For this review, take the finished solid that the model builds, in its own axes (mm). Face numbers are marked on the shaded views. Round coordinates to 2 decimals unless told otherwise and drop trailing zeros. Loops run counter-clockwise (first coordinate to the right, second up) from the corner with the lowest first, then second, coordinate; pieces in that order, holes last.
1. Consider section C-C on x = -25. State the section outline as (y, z) points.
2. Consider section D-D on y = 0.4. State the section outline as (x, z) points.
3. To check wall thickness, follow line 1 along Z through (x, y) = (-12.25, 2.3); line 2 along X through (y, z) = (1.45, -5); line 3 along Y through (x, z) = (-22.25, -6.5). State the ranges of each line that lie inside material, in increasing order.
4. Consider section B-B on z = 9.5. State the section outline as (x, y) points.
5. Consider section A-A on y = 1.7. State the section outline as (x, z) points, then the cut area to 3 significant figures.
6. Draft analysis for pull direction X (two halves, no side actions). For the marked faces 1, 2, 3 and 4, state which applies: released by +X, released by -X, zero draft, split by the parting line, or undercut.
7. Clearance check with flat-ended pins moving along their axes: pin 1 Ø2 at (x, z) = (-14.5, 2) entering from +Y; pin 2 Ø1.1 at (x, y) = (-19.5, 0.5) entering from +Z. State where each tip first meets the part, or that it passes through.
from build123d import *

# Parameters (mm, degrees)
MAIN_BOARD_OUTLINE_W = 18.5
MAIN_BOARD_OUTLINE_H = 28
SIDE1_DEPTH          = 1
SKETCH2_W            = 2
SKETCH2_H            = 28
WALLS_DEPTH          = 2.3
SKETCH3_R            = 1.5
SCREW_HOLE_DEPTH     = 2.3
SKETCH4_W            = 4.6228
SKETCH4_H            = 2
SPI_HOLE_DEPTH       = 2.3
SKETCH5_W            = 2
SKETCH5_H            = 4
CUT_EXTRUDE3_DEPTH   = 2.3


with BuildPart() as part:
    # main board outline → side1 (new body)
    with BuildSketch(Plane(origin=(0, 0, 0), x_dir=(1, 0, 0), z_dir=(0, 1, 0))):
        with Locations((-19.997374583, 0.651042113)):
            Rectangle(MAIN_BOARD_OUTLINE_W, MAIN_BOARD_OUTLINE_H)
    extrude(amount=SIDE1_DEPTH)

    # Sketch2 → walls (add)
    with BuildSketch(Plane(origin=(0, 1, 0), x_dir=(1, 0, 0), z_dir=(0, 1, 0))):
        with Locations((-28.247374583, 0.651042113)):
            Rectangle(SKETCH2_W, SKETCH2_H)
        with Locations((-11.747374583, 0.651042113)):
            Rectangle(SKETCH2_W, SKETCH2_H)
    extrude(amount=WALLS_DEPTH)

    # Sketch3 → screw hole (cut)
    with BuildSketch(Plane(origin=(0, 0, 0), x_dir=(-1, 0, 0), z_dir=(0, -1, 0))):
        with Locations((24.504374583, -10.605757887)):
            Circle(SKETCH3_R)
    extrude(amount=-SCREW_HOLE_DEPTH, mode=Mode.SUBTRACT)

    # Sketch4 → spi hole (cut)
    with BuildSketch(Plane(origin=(0, 0, 0), x_dir=(-1, 0, 0), z_dir=(0, -1, 0))):
        with Locations((18.687974583, -12.348957887)):
            Rectangle(SKETCH4_W, SKETCH4_H)
    extrude(amount=-SPI_HOLE_DEPTH, mode=Mode.SUBTRACT)

    # Sketch5 → Cut-Extrude3 (cut)
    with BuildSketch(Plane(origin=(0, 3.3, 0), x_dir=(1, 0, 0), z_dir=(0, 1, 0))):
        with Locations((-28.247374583, 8.651042113)):
            Rectangle(SKETCH5_W, SKETCH5_H)
        with Locations((-28.247374583, -4.348957887)):
            Rectangle(SKETCH5_W, SKETCH5_H)
        with Locations((-11.747374583, 8.651042113)):
            Rectangle(SKETCH5_W, SKETCH5_H)
        with Locations((-11.747374583, -4.348957887)):
            Rectangle(SKETCH5_W, SKETCH5_H)
    extrude(amount=-CUT_EXTRUDE3_DEPTH, mode=Mode.SUBTRACT)


solid = part.part
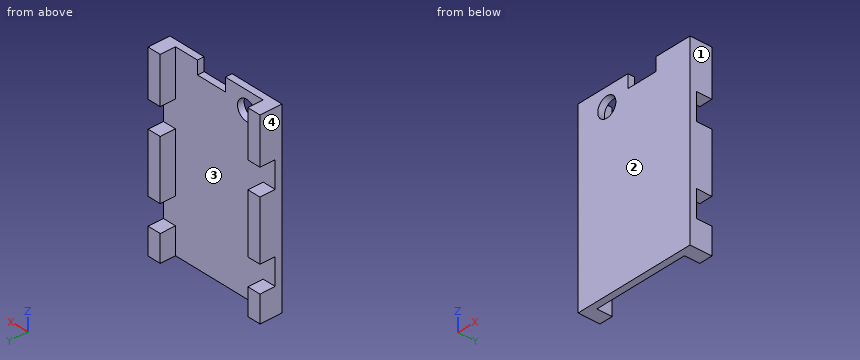
Resolved:
1. outline: (0, -14.65) - (1, -14.65) - (1, 9.19) - (0, 9.19) - close; (0, 12.02) - (1, 12.02) - (1, 13.35) - (0, 13.35) - close
2. outline: (-29.25, -14.65) - (-10.75, -14.65) - (-10.75, 13.35) - (-16.38, 13.35) - (-16.38, 11.35) - (-21, 11.35) - (-21, 13.35) - (-29.25, 13.35) - close; hole circle Ø3 at (-24.5, 10.61)
3. line 1: z = -14.65 to -10.65, -6.65 to 2.35, 6.35 to 13.35
3. line 2: x = -29.25 to -27.25, -12.75 to -10.75
3. line 3: y = 0 to 1
4. outline: (-29.25, 0) - (-25.52, 0) - (-25.52, 1) - (-27.25, 1) - (-27.25, 3.3) - (-29.25, 3.3) - close; (-23.49, 0) - (-10.75, 0) - (-10.75, 3.3) - (-12.75, 3.3) - (-12.75, 1) - (-23.49, 1) - close
5. outline: (-29.25, -14.65) - (-27.25, -14.65) - (-27.25, -10.65) - (-29.25, -10.65) - close; (-29.25, -6.65) - (-27.25, -6.65) - (-27.25, 2.35) - (-29.25, 2.35) - close; (-29.25, 6.35) - (-27.25, 6.35) - (-27.25, 13.35) - (-29.25, 13.35) - close; (-12.75, -14.65) - (-10.75, -14.65) - (-10.75, -10.65) - (-12.75, -10.65) - close; (-12.75, -6.65) - (-10.75, -6.65) - (-10.75, 2.35) - (-12.75, 2.35) - close; (-12.75, 6.35) - (-10.75, 6.35) - (-10.75, 13.35) - (-12.75, 13.35) - close
5. area: 80.0 mm2
6. face 1: released by +X
6. face 2: zero draft
6. face 3: undercut
6. face 4: released by -X
7. pin 1: stops at y = 1
7. pin 2: stops at z = 11.35
